Check sheet for the drawn part. Datum: minimum x, y, z corner. Units: mm. Round coordinates to 2 decimals unless told otherwise and drop trailing zeros. Order: outer loops, then holes, each group sorted by start corner. A loop starts at its lowest first (then second) coordinate and runs counter-clockwise, first axis right, second up. Notation, with made-up numbers: M 2,15 L 25,15 A33 cw 25,44 Z; hole C -32.5,56 d4. An arc over 180 degrees is marked long. Use one line per item in the form item = value. Start each with the question number.
Item 1: Thickness scan on probe 1 along X at (y, z) = (5.5, 9). Record the ranges inside material, lowest first. Write a range as [from, to].
Item 2: Go/stop test with a flat-tipped pin: pin 1 Ø3 at (x, y) = (38.5, 1.5) entering from -Z. Record where the tip stops, or that it passes through.
Item 3: Cross-section at A-A on x = 60. Enter the section's corners in (y, z), then the cut area to 3 significant figures.
Item 4: Cross-section at C-C on x = 71.5. Enter the section's corners in (y, z), then the cut area to 3 significant figures.
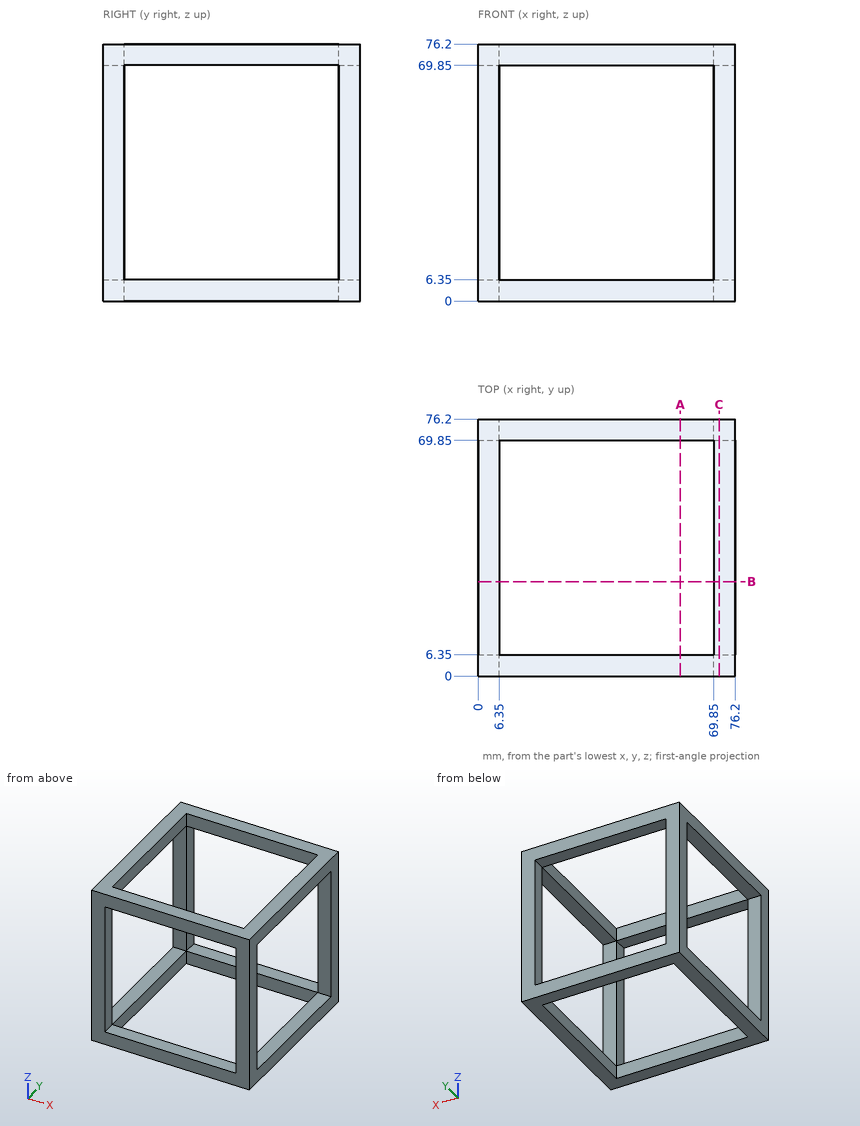
Output values:
q1.probe_1 = [0, 6.35], [69.85, 76.2]
q2.pin_1 = 0
q3.outline = M 0,0 L 6.35,0 L 6.35,6.35 L 0,6.35 Z; M 0,69.85 L 6.35,69.85 L 6.35,76.2 L 0,76.2 Z; M 69.85,0 L 76.2,0 L 76.2,6.35 L 69.85,6.35 Z; M 69.85,69.85 L 76.2,69.85 L 76.2,76.2 L 69.85,76.2 Z
q3.area = 161 mm2
q4.outline = M 0,0 L 76.2,0 L 76.2,76.2 L 0,76.2 Z; hole M 6.35,6.35 L 69.85,6.35 L 69.85,69.85 L 6.35,69.85 Z
q4.area = 1,770 mm2
